Could you check a few things on this model? Use its own coordinates, in mm. Face numbers are marked on the shaded views. A direction names the side the tool comes from. Coordinates: 2 decimals unless noted, no trailing zeros. Order: outer loops, then holes, each group sorted by start corner. A loop starts at its lowest first (then second) coordinate and runs counter-clockwise, first axis right, second up. Notation, with made-up numbers: (54, 51) -> (105, 51) arc R13 cw to (105, 66) -> close; hole circle Ø4 at (50.25, 12.5). An arc over 180 degrees is marked (long way). Return JSON: item names as keys, results as strings. Group by question number.
from build123d import *

# Parameters (mm, degrees)
PAD030_DEPTH            = 19
SKETCH090_W             = 9
SKETCH090_H             = 27
POCKET054_DEPTH         = 15
SKETCH089_R             = 1.6
POCKET053_DEPTH         = 5
CHAMFER010_SIZE         = 0.3
BODY020_PLACEMENT_ANGLE = 22.5


with BuildPart() as part:
    # Sketch088 → Pad030 (new body)
    with BuildSketch(Plane.YZ):
        with BuildLine():
            ThreePointArc((11.6189500386, 3), (0, 12), (-11.6189500386, 3))
            Line((-11.6189500386, 3), (-14, -41))
            Line((-24, -41), (-14, -41))
            Line((-24, -45), (-24, -41))
            Line((24, -45), (-24, -45))
            Line((24, -41), (24, -45))
            Line((14, -41), (24, -41))
            Line((14, -41), (11.6189500386, 3))
        make_face()
        Polygon((7.6210235533, 3.5), (3.8105117767, 10.1), (-3.8105117767, 10.1), (-7.6210235533, 3.5), (-3.8105117767, -3.1), (3.8105117767, -3.1), align=None, mode=Mode.SUBTRACT)
    extrude(amount=PAD030_DEPTH)

    # Sketch090 → Pocket054 (cut, symmetric)
    with BuildSketch(Plane.XZ):
        with Locations((9.5, 1.5)):
            Rectangle(SKETCH090_W, SKETCH090_H)
    extrude(amount=POCKET054_DEPTH, both=True, mode=Mode.SUBTRACT)

    # Sketch089 (on Face8 of Pocket054) → Pocket053 (cut)
    with BuildSketch(Plane.YX.offset(45)):
        with Locations((-18, 9.5)):
            Circle(SKETCH089_R)
        with Locations((18, 9.5)):
            Circle(SKETCH089_R)
    extrude(amount=-POCKET053_DEPTH, mode=Mode.SUBTRACT)

    # Chamfer010
    chamfer010_edges = [part.edges().sort_by_distance(p)[0] for p in [
        (9.5, 16.4, -41),
        (9.5, -19.6, -41),
        (9.5, -24, -41),
        (9.5, 24, -41),
    ]]
    chamfer(chamfer010_edges, length=CHAMFER010_SIZE)


with BuildPart() as part_1:
    # Body020 placement: moved
    add(part.part.moved(Location((74.8148666983, -31.0129027885, 55.1))).rotate(Axis((74.8148666983, -31.0129027885, 55.1), (0, 0, -1)), BODY020_PLACEMENT_ANGLE))


solid = part_1.part
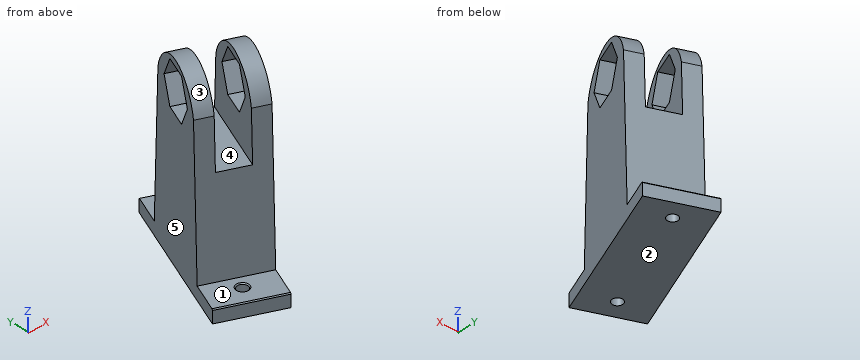
Q1. We'd pull the mould along X, two halves only. Please class the marked faces 3, 4 and 5: pulls with the +X half, pulls with the -X half, needs draft (parallel to the pull), parting line crosses it, or undercut.
Q2. I want a section at A-A on z = 56. Please give me the cut outline in (x, y) (3 decimals), and give its area (3 significant figures).
Q3. On a 3-axis mill with a long thin cutter (end or side, diameter ignored), from which of +Z, -Z, +X, -X, +Y, -Y can I reach the whole of each face in a straight line? I mean the marked faces 1 and 2. Say none if no direction works.
Q4. I need wall thicknesses on line 1 along Z through (x, y) = (67, -50.5); line 2 along Z through (x, y) = (85, -37); line 3 along X through (y, z) = (-25.5, 26.5). Which ranges of each line are inside material? Lowest first, please. Write a range as from..to.
Q5. I want a section at C-C on x = 99. Please give me the cut outline in (y, z), and give its area (3 significant figures).
Q6. I want a section at B-B on z = 49. Please give me the cut outline in (x, y), and give its area (3 significant figures).
Q7. I'm going to push flat-ended pins straight in: pin 1 Ø8 at (x, z) = (88.5, 44) entering from +Y; pin 2 Ø6 at (y, z) = (-39, 18.5) entering from +X; pin 3 Ø2 at (y, z) = (-28, 36) entering from +X. Where does each tip first touch, or does it pass through?
Q8. I want a section at D-D on z = 30.5. Please give me the cut outline in (x, y), and give its area (3 significant figures).
Response values:
{
 "1": {"face 3": "parting line crosses it", "face 4": "undercut", "face 5": "pulls with the -X half"},
 "2": {"outline": "(70.325, -41.852) -> (74.944, -43.766) -> (77.092, -38.58) -> (72.473, -36.667) -> close; (77.157, -25.359) -> (81.776, -27.272) -> (83.924, -22.087) -> (79.305, -20.173) -> close; (83.259, -47.21) -> (87.879, -49.123) -> (90.027, -43.938) -> (85.407, -42.025) -> close; (90.091, -30.716) -> (94.711, -32.63) -> (96.858, -27.444) -> (92.239, -25.531) -> close", "area": "112 mm²"},
 "3": {"face 1": "+Z, -X, -Y", "face 2": "-Z, +X, -X, +Y, -Y"},
 "4": {"line 1": "z = 10.1..14.1", "line 2": "z = 10.1..43.1", "line 3": "x = 77.1..96.34"},
 "5": {"outline": "(-22.27, 10.1) -> (-15.05, 10.1) -> (-15.05, 13.8) -> (-15.38, 14.1) -> (-22.27, 14.1) -> close", "area": "28.8 mm²"},
 "6": {"outline": "(70.18, -42.2) -> (74.8, -44.12) -> (84.07, -21.74) -> (79.45, -19.82) -> close; (83.11, -47.56) -> (87.73, -49.47) -> (97, -27.09) -> (92.38, -25.18) -> close", "area": "242 mm²"},
 "7": {"pin 1": "stops at y = -21.61", "pin 2": "stops at x = 93.31", "pin 3": "stops at x = 97.04"},
 "8": {"outline": "(69.8, -43.13) -> (87.35, -50.4) -> (97.39, -26.17) -> (79.83, -18.9) -> close", "area": "498 mm²"}
}
